Source: CAD feature listing. Evaluate the final solid. Frame: model axes, mm. Round coordinates to 2 decimals unless told otherwise and drop trailing zeros. Loops run counter-clockwise (first coordinate to the right, second up) from the corner with the lowest first, then second, coordinate; pieces in that order, holes last. Notation, with made-up numbers: M -38.5,2 L 5.5,2 A8 ccw 5.5,13 Z; hole C 40,-12.5 d5. An arc over 180 degrees is marked long. Answer as CSV lines item,"result". Start each with the question number.
Autodesk Inventor part; units mm, degrees
ref_plane "YZ Plane" through (0, 0, 0) normal (1, 0, 0) x (0, 1, 0)
ref_plane "XZ Plane" through (0, 0, 0) normal (0, 1, 0) x (-1, 0, 0)
ref_plane "XY Plane" through (0, 0, 0) normal (0, 0, 1) x (1, 0, 0)
sketch "Sketch1" plane through (0, 0, 0) normal (0, 0, 1) x (1, 0, 0)
  circle A0 centre (0, 0) radius 1
  circle A1 centre (-14, 0) radius 1
  line L0 (-14, 2) -> (16, 2)
  line L1 (16, -2) -> (-14, -2)
  arc A2 (-14, 2) -> (-14, -2) centre (-14, 0) ccw
  circle A3 centre (16, 0) radius 1
  arc A4 (16, -2) -> (16, 2) centre (16, 0) ccw
  dimension "d0" = 2
  dimension "d1" = 14
  dimension "d5" = 16
  dimension "d6" = 2
extrude "Extrusion1" add sketch "Sketch1" along normal blind 2
properties part number "panto_linkageC"
1) Section C-C, the plane x = 0. Return loops of the section in (y, z), and give its area (3 significant figures).
2) Section B-B, the plane z = 1.45. Return loops of the section in (x, y).
3) Section D-D, the plane y = -1.4. Return loops of the section in (x, z), and give its area (3 significant figures).
4) Contact query for a flat-ended pin moving along its axis: pin 1 Ø1.8 at (x, y) = (16, 0) entering from -Z. Output: stop coordinate, or through.
5) Section A-A, the plane y = 0. Return loops of the section in (x, z), and give its area (3 significant figures).
6) Mould query, pull axis X, two halves, no side actions, for faces 1 (the flat face through (1, 1, 0)), 2 (the cylindrical face through (-16, 0, 1)), 3 (the cylindrical face through (-13, 0, 1)), 4 (the cylindrical face through (17, 0, 1)). Classes: pulls with the +X half, pulls with the -X half, needs draft (parallel to the pull), parting line crosses it, or undercut.
7) Ray query, line 1 along X through (y, z) = (-0.15, 1.1); line 2 along Y through (x, z) = (-14, 1.1); line 3 along X through (y, z) = (-1.8, 0.75). Return the intervals inside material, ascending.
Findings below:
1,outline,"M -2,0 L -1,0 L -1,2 L -2,2 Z; M 1,0 L 2,0 L 2,2 L 1,2 Z"
1,area,"4.00 mm²"
2,outline,"M -14,-2 L 16,-2 A2 ccw 16,2 L -14,2 A2 ccw Z; hole C -14,0 d2; hole C 0,0 d2; hole C 16,0 d2"
3,outline,"M -15.43,0 L 17.43,0 L 17.43,2 L -15.43,2 Z"
3,area,"65.7 mm²"
4,pin 1,"through"
5,outline,"M -16,0 L -15,0 L -15,2 L -16,2 Z; M -13,0 L -1,0 L -1,2 L -13,2 Z; M 1,0 L 15,0 L 15,2 L 1,2 Z; M 17,0 L 18,0 L 18,2 L 17,2 Z"
5,area,"56.0 mm²"
6,face 1,"needs draft"
6,face 2,"pulls with the -X half"
6,face 3,"undercut"
6,face 4,"undercut"
7,line 1,"-15.99 to -14.99, -13.01 to -0.99, 0.99 to 15.01, 16.99 to 17.99"
7,line 2,"-2 to -1, 1 to 2"
7,line 3,"-14.87 to 16.87"
